CAD build for the part. Positions are in the model's coordinates, mm. A direction names the side the tool comes from. Coordinates: 2 decimals unless noted, no trailing zeros. Order: outer loops, then holes, each group sorted by start corner. A loop starts at its lowest first (then second) coordinate and runs counter-clockwise, first axis right, second up. Notation, with made-up numbers: M -28,-6 L -2,-6 A14 cw -2,19 Z; hole C 57,75.25 d9. An arc over 180 degrees is marked long. Write item = value, one per line. Start each with the question number.
Autodesk Inventor part; units mm, degrees
ref_plane "YZ Plane" through (0, 0, 0) normal (1, 0, 0) x (0, 1, 0)
ref_plane "XZ Plane" through (0, 0, 0) normal (0, 1, 0) x (-1, 0, 0)
ref_plane "XY Plane" through (0, 0, 0) normal (0, 0, 1) x (1, 0, 0)
sketch "Эскиз1" plane through (0, 0, 0) normal (1, 0, 0) x (0, 1, 0)
  line L0 (-50, -978) -> (50, -978)
  line L1 (50, -978) -> (50, 978)
  line L2 (50, 978) -> (-50, 978)
  line L3 (-50, 978) -> (-50, -978)
  line L4 (-50, -978) -> (50, 978) construction
  line L5 (50, -978) -> (-50, 978) construction
  point P0 (0, 0)
  dimension "d0" = 100
  dimension "d1" = 1956
extrude "Выдавливание1" add sketch "Эскиз1" along normal blind 50
sketch "Эскиз2" plane through (0, 50, 978) normal (0, 1, 0) x (1, 0, 0)
  line L0 (0, 1556) -> (10, 1556)
  line L1 (10, 1463) -> (0, 1463)
  line L2 (10, 1463) -> (10, 1556)
  line L3 (0, 1556) -> (0, 1463)
  point P0 (0, 978)
extrude "Выдавливание2" cut sketch "Эскиз2" against normal blind 55
sketch "Эскиз3" plane through (0, 50, 978) normal (0, 1, 0) x (1, 0, 0)
  line L0 (10, 493) -> (-0.0484, 493)
  line L1 (0, 400) -> (10, 400)
  line L2 (10, 400) -> (10, 493)
  line L3 (-0.0484, 493) -> (0, 400)
  point P0 (0, 978)
extrude "Выдавливание3" cut sketch "Эскиз3" against normal blind 29
properties part number "side_panel"
1. 3-axis set-ups, long thin cutter, end or side, ignore diameter. For faces 1 (the flat face through (10, 23, -531)), 2 (the flat face through (25, -50, 14)): which of +Z, -Z, +X, -X, +Y, -Y reach the whole face in a straight line?
2. Slice it at A-A (z = -516). Write the cut outline in (x, y), plus the area to 3 significant figures.
3. Flat gauge pins, fed straight in: pin 1 (14.5 mm diameter, centred on y = 28.5, z = 544.5, fed in from -X); pin 2 (8 mm diameter, centred on x = 5.5, z = 527, fed in from +Y). Where does each tip first touch, or does it go through?
Calculated:
q1.face_1 = -X, +Y
q1.face_2 = +Z, -Z, +X, -X, -Y
q2.outline = M 0,-50 L 50,-50 L 50,50 L 10,50 L 10,-5 L 0,-5 Z
q2.area = 4,450 mm²
q3.pin_1 = 10
q3.pin_2 = 21
